```python
from build123d import *

# Parameters (mm, degrees)
F0_R     = 2.2
F0_R_2   = 2.1971
F1_DEPTH = 7.62
F2_W     = 8.5971400267
F2_H     = 2.54
F2_W_2   = 43.3469019601
F3_DEPTH = 12.7
F5_DEPTH = 25.4


with BuildPart() as f1:
    # F0 (on Top) → F1 (new body)
    with BuildSketch(Plane.XY):
        with BuildLine():
            Line((5.9369556572, -27.8083572605), (39.6794228829, -27.9006065895))
            Line((39.6794228829, -27.9006065895), (55.7396312141, -15.4518271971))
            ThreePointArc((55.7396312141, -15.4518271971), (54.6110684248, -6.7600664581), (47.5776399311, -11.9899079794))
            ThreePointArc((47.5776399311, -11.9899079794), (47.1582083615, -15.0471734784), (45.347095709, -17.5457062744))
            Line((45.347095709, -17.5457062744), (39.2019450665, -22.7020999121))
            Line((39.2019450665, -22.7020999121), (5.8364926789, -22.7020999121))
            ThreePointArc((5.8364926789, -22.7020999121), (2.8430739719, -21.9522735206), (0.5565983665, -19.8798776899))
            ThreePointArc((0.5565983665, -19.8798776899), (-8.1474559702, -20.3073649465), (-3.6673170835, -27.7820999121))
            Line((-3.6673170835, -27.7820999121), (5.9369556572, -27.8083572605))
        make_face()
        with Locations((-3.6673170835, -22.7020999121)):
            Circle(F0_R, mode=Mode.SUBTRACT)
        with Locations((52.627436366, -11.4367751143)):
            Circle(F0_R_2, mode=Mode.SUBTRACT)
    extrude(amount=F1_DEPTH)

    # F2 (on face) → F3 (cut, symmetric)
    with BuildSketch(Plane(origin=(-0.0759809827, -27.7919183508, 0), x_dir=(0.9999962629, -0.0027339134, 0), z_dir=(-0.0027339134, -0.9999962629, 0))):
        with Locations((-7.8899195355, 1.27)):
            Rectangle(F2_W, F2_H)
        with Locations((18.0821014579, 1.27)):
            Rectangle(F2_W_2, F2_H)
        with Locations((-7.8899195355, 6.35)):
            Rectangle(F2_W, F2_H)
        with Locations((18.0821014579, 6.35)):
            Rectangle(F2_W_2, F2_H)
    extrude(amount=F3_DEPTH, both=True, mode=Mode.SUBTRACT)

    # F4 (on face) → F5 (cut)
    with BuildSketch(Plane(origin=(28.4022854633, -36.6418752591, 0), x_dir=(0.7903645832, 0.6126367811, 0), z_dir=(0.6126367811, -0.7903645832, 0))):
        with BuildLine():
            Line((14.2682727173, 5.08), (15.6822027681, 5.08))
            ThreePointArc((15.6822027681, 5.08), (22.0769997922, 5.8758387603), (28.2806027681, 7.62))
            Line((28.2806027681, 7.62), (14.2682727173, 7.62))
            Line((14.2682727173, 7.62), (14.2682727173, 5.08))
        make_face()
        Polygon((34.5882727173, 2.04), (34.5882727173, 5.58), (29.5646376908, 5.58), (29.5646376908, 5.08), (29.5646376908, 4.3004048057), (29.5646376908, 3.3195951943), (29.5646376908, 2.54), (29.5646376908, 2.04), align=None)
        Polygon((41.6956804693, 5.58), (34.5882727173, 5.58), (34.5882727173, 2.04), (41.6956804693, 2.04), (42.2389656305, 2.04), (42.2389656305, 2.54), (42.2389656305, 3.4030259121), (42.2389656305, 4.2169740879), (42.2389656305, 5.08), (42.2389656305, 5.58), align=None)
        with BuildLine():
            Line((15.6822027681, 2.54), (14.2682727173, 2.54))
            Line((14.2682727173, 2.54), (14.2682727173, 0))
            Line((14.2682727173, 0), (28.2806027681, 0))
            ThreePointArc((28.2806027681, 0), (22.0769997922, 1.7441612397), (15.6822027681, 2.54))
        make_face()
    extrude(amount=-F5_DEPTH, mode=Mode.SUBTRACT)


solid = f1.part
```
Read the model definition and answer for the solid it produces. Units are mm, in the model's axes. A direction names the side the tool comes from. Give positions to 0.01 mm unless a question says otherwise; leave off trailing zeros. Write each loop counter-clockwise with the first axis right and the second up, starting at its lowest first coordinate (ties: lowest second). Pieces come first, ordered by that corner, then holes. Notation, with made-up numbers: (57, 13) -> (98, 13) arc R18 ccw to (98, 27) -> close; hole circle Ø7 at (46.25, 71). An arc over 180 degrees is marked (long way). Answer in a Markdown table with one row per item.
1) Section D-D on x = 18 is taken. Give the vertices of the cut face in (y, z), plus the area to 3 significant figures.
Results list:
| item | result |
|---|---|
| outline | (-27.84, 2.54) -> (-22.7, 2.54) -> (-22.7, 5.08) -> (-27.84, 5.08) -> close |
| area | 13.1 mm^2 |
2) Determine the mould class of faces 1 (the flat face through (47.6, -21.76, 3.76)), 2 (the flat face through (52, -14, 5.58)), 3 (the cylindrical face through (44.584, -21.337, 1.726)), 4 (the flat face through (14, -24, 5.08)) for opening direction Z: released by +Z, released by -Z, zero draft, split by the parting line, or undercut.
Results list:
| item | result |
|---|---|
| face 1 | zero draft |
| face 2 | undercut |
| face 3 | released by -Z |
| face 4 | released by +Z |
3) Section C-C on x = 52.5 is taken. Give the vertices of the cut face in (y, z).
Results list:
| item | result |
|---|---|
| outline | (-17.96, 0) -> (-13.63, 0) -> (-13.63, 2.04) -> (-17.96, 2.04) -> close; (-17.96, 5.58) -> (-13.63, 5.58) -> (-13.63, 7.62) -> (-17.96, 7.62) -> close; (-9.24, 0) -> (-6.36, 0) -> (-6.36, 2.04) -> (-9.24, 2.04) -> close; (-9.24, 5.58) -> (-6.36, 5.58) -> (-6.36, 7.62) -> (-9.24, 7.62) -> close |
4) Section A-A on z = 4.5 is taken. Give the vertices of the cut face in (x, y), plus the area to 3 significant figures.
Results list:
| item | result |
|---|---|
| outline | (-3.67, -27.78) -> (39.68, -27.9) -> (51.77, -18.53) -> (47.6, -13.15) arc R6.35 cw to (45.35, -17.55) -> (39.2, -22.7) -> (5.84, -22.7) arc R6.35 cw to (0.56, -19.88) arc R5.08 ccw (long way) to start; hole circle Ø4.4 at (-3.67, -22.7) |
| area | 337 mm^2 |
5) Straight lines are drawn through the part: line 1 (X direction, y = -21.75, z = 3.75); line 2 (Y direction, x = 35, z = 3.75); line 3 (X direction, y = -10, z = 7.5). For each, find the intervals that lie inside material, in ascending order. Write a range as [from, to].
Results list:
| item | result |
|---|---|
| line 1 | [-8.66, -5.65], [-1.68, 2.49], [40.34, 47.61] |
| line 2 | [-27.89, -22.7] |
| line 3 | [47.75, 50.97], [54.29, 57.5] |
6) Section B-B on y = -8.25 is taken. Give the vertices of the cut face in (x, z).
Results list:
| item | result |
|---|---|
| outline | (48.67, 0) -> (56.58, 0) -> (56.58, 2.04) -> (48.67, 2.04) -> close; (48.67, 5.58) -> (56.58, 5.58) -> (56.58, 7.62) -> (48.67, 7.62) -> close |
7) A tool of negligible diameter and unlimited length cuts with its end or side. For faces 5 (the cylindrical face through (50.432, -11.34, 6.586)), 6 (the flat face through (52, -14, 2.04)), 7 (the flat face through (23, -22.702, 4)), from which of +Z, -Z, +X, -X, +Y, -Y can it reach the whole face along a straight path? Write none if from no direction.
Results list:
| item | result |
|---|---|
| face 5 | +Z, -Z |
| face 6 | +X, +Y |
| face 7 | +Z, -Z, +Y |
8) Each of these flat-tipped pins is pushed along its axis until it touches: pin 1 Ø10 at (x, y) = (35.5, -22) entering from +Z; pin 2 Ø12 at (x, y) = (-2, -21.5) entering from +Z; pin 3 Ø3 at (x, z) = (25.5, 2) entering from -Y. Where does it stop, or does it pass through?
Results list:
| item | result |
|---|---|
| pin 1 | z = 5.34 |
| pin 2 | z = 5.08 |
| pin 3 | y = -27.87 |
